```python
from build123d import *

# Parameters (mm, degrees)
F0_R     = 6.35
F0_R_2   = 5.842
F1_DEPTH = 50.8
F0_W     = 81.28
F0_H     = 15.24
F2_DEPTH = 1.27


with BuildPart() as f1:
    # F0 (on Top) → F1 (new body)
    with BuildSketch(Plane.XY):
        with Locations((-31.75, 0)):
            Circle(F0_R)
        with Locations((-31.75, 0)):
            Circle(F0_R_2, mode=Mode.SUBTRACT)
    extrude(amount=F1_DEPTH)



with BuildPart() as f1b:
    # F0 (on Top) → F1, piece 2 (new body)
    with BuildSketch(Plane.XY):
        with Locations((31.75, 0)):
            Circle(F0_R)
        with Locations((31.75, 0)):
            Circle(F0_R_2, mode=Mode.SUBTRACT)
    extrude(amount=F1_DEPTH)


with BuildPart() as f1_1:
    add(f1.part)

    add(f1b.part)  # F2 merges F1b
    # F0 (on Top) → F2 (join)
    with BuildSketch(Plane.XY):
        Rectangle(F0_W, F0_H)
        with Locations((-31.75, 0)):
            Circle(F0_R, mode=Mode.SUBTRACT)
        with Locations((31.75, 0)):
            Circle(F0_R, mode=Mode.SUBTRACT)
    extrude(amount=F2_DEPTH)


solid = f1_1.part
```
For this review, take the finished solid that the model builds, in its own axes (mm). A direction names the side the tool comes from. Round coordinates to 2 decimals unless told otherwise and drop trailing zeros. Loops run counter-clockwise (first coordinate to the right, second up) from the corner with the lowest first, then second, coordinate; pieces in that order, holes last.
(1) Wall thickness on line 1 along X through (y, z) = (0.25, 12); line 2 along X through (y, z) = (2.5, 7.5); line 3 along Y through (x, z) = (-31.75, 26): over which ranges is each line inside the solid? List them lowest first.
Returned:
line 1: x = -38.1 to -37.59, -25.91 to -25.4, 25.4 to 25.91, 37.59 to 38.1
line 2: x = -37.59 to -37.03, -26.47 to -25.91, 25.91 to 26.47, 37.03 to 37.59
line 3: y = -6.35 to -5.84, 5.84 to 6.35
(2) We need section D-D (y = 4.25). Give the boundary of the cut face in (x, z), plus the area to 3 significant figures.
Returned:
outline: (-40.64, 0) - (-35.76, 0) - (-35.76, 50.8) - (-36.47, 50.8) - (-36.47, 1.27) - (-40.64, 1.27) - close; (-27.74, 0) - (27.74, 0) - (27.74, 50.8) - (27.03, 50.8) - (27.03, 1.27) - (-27.03, 1.27) - (-27.03, 50.8) - (-27.74, 50.8) - close; (35.76, 0) - (40.64, 0) - (40.64, 1.27) - (36.47, 1.27) - (36.47, 50.8) - (35.76, 50.8) - close
area: 223 mm2
(3) We need section B-B (x = 31.75). Give the boundary of the cut face in (y, z).
Returned:
outline: (-7.62, 0) - (-5.84, 0) - (-5.84, 50.8) - (-6.35, 50.8) - (-6.35, 1.27) - (-7.62, 1.27) - close; (5.84, 0) - (7.62, 0) - (7.62, 1.27) - (6.35, 1.27) - (6.35, 50.8) - (5.84, 50.8) - close
(4) Mouldability with a two-part tool opening along Y and no side actions: class faces 1 (the cylindrical face through (-25.693, 1.907, 25.688)), 2 (the flat face through (37, -3, 50.8)), 3 (the cylindrical face through (37.322, 1.755, 25.044)) as released by +Y, released by -Y, zero draft, split by the parting line, or undercut.
Returned:
face 1: split by the parting line
face 2: zero draft
face 3: undercut
(5) We need section A-A (y = 0). Give the boundary of the cut face in (x, z), plus the area to 3 significant figures.
Returned:
outline: (-40.64, 0) - (-37.59, 0) - (-37.59, 50.8) - (-38.1, 50.8) - (-38.1, 1.27) - (-40.64, 1.27) - close; (-25.91, 0) - (25.91, 0) - (25.91, 50.8) - (25.4, 50.8) - (25.4, 1.27) - (-25.4, 1.27) - (-25.4, 50.8) - (-25.91, 50.8) - close; (37.59, 0) - (40.64, 0) - (40.64, 1.27) - (38.1, 1.27) - (38.1, 50.8) - (37.59, 50.8) - close
area: 174 mm2
(6) Tool access review of faces 4 (the cylindrical face through (-26.353, -2.238, 25.044)), 5 (the cylindrical face through (37.807, 1.907, 25.688)): name each direction out of +Z, -Z, +X, -X, +Y, -Y from which nothing blocks a thin tool from reaching the whole face with its end or side.
Returned:
face 4: +Z, -Z
face 5: +Z
(7) We need section C-C (z = 13). Give the boundary of the cut face in (x, y), plus the area to 3 significant figures.
Returned:
outline: circle Ø12.7 at (-31.75, 0); circle Ø12.7 at (31.75, 0); hole circle Ø11.68 at (-31.75, 0); hole circle Ø11.68 at (31.75, 0)
area: 38.9 mm2
(8) Clearance check with flat-ended pins moving along their axes: P1, Ø3, axis at x = -25, y = -4.5, coming from the +Z side; P2, Ø5, axis at y = -1, z = 14, coming from the +X side; P3, Ø3, axis at x = 31.5, z = 15.5, coming from the +Y side; P4, Ø4, axis at x = -22, y = -1, coming from the -Z side. State where each tip first meets the part, or that it passes through.
Returned:
P1: stops at z = 1.27
P2: stops at x = 38.1
P3: stops at y = 6.35
P4: stops at z = 0
